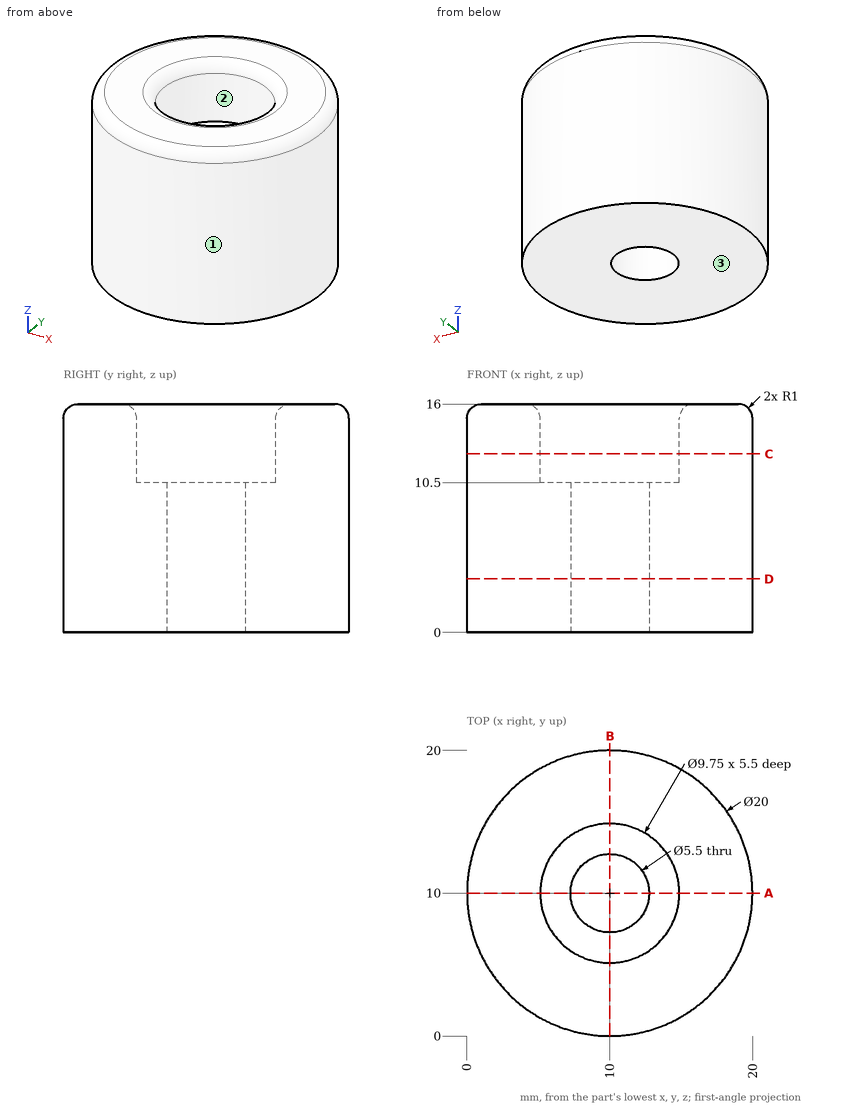
Here's the drawing with two shaded views (mm, measured from the low corner). I have some questions. Coordinates: 2 decimals unless noted, no trailing zeros. Order: outer loops, then holes, each group sorted by start corner. A loop starts at its lowest first (then second) coordinate and runs counter-clockwise, first axis right, second up. Notation, with made-up numbers: (70.5, 51) -> (86.5, 51) arc R19 ccw to (86.5, 85) -> close; hole circle Ø11 at (5, 29.25). An arc over 180 degrees is marked (long way). Write each question's results on one line, items separated by ' | '.
Item 1: I want a section at D-D, the plane z = 3.75. Write out the boundary of the cut face in (x, y), then the cut area to 3 significant figures.
Results are:
outline: circle Ø20 at (10, 10); hole circle Ø5.5 at (10, 10) | area: 290 mm²
Item 2: I want a section at C-C, the plane z = 12.5. Write out the boundary of the cut face in (x, y) (3 decimals), then the cut area to 3 significant figures.
Results are:
outline: circle Ø20 at (10, 10); hole circle Ø9.75 at (10, 10) | area: 239 mm²
Item 3: I want a section at A-A, the plane y = 10. Write out the boundary of the cut face in (x, z) (3 decimals).
Results are:
outline: (0, 0) -> (7.25, 0) -> (7.25, 10.5) -> (5.125, 10.5) -> (5.125, 15) arc R1 ccw to (4.125, 16) -> (1, 16) arc R1 ccw to (0, 15) -> close; (12.75, 0) -> (20, 0) -> (20, 15) arc R1 ccw to (19, 16) -> (15.875, 16) arc R1 ccw to (14.875, 15) -> (14.875, 10.5) -> (12.75, 10.5) -> close
Item 4: If we mould it in two halves opening along Y, with no side actions, what happens to the marked faces 1, 2 and 3? For each: +Y half, -Y half, draft (parallel to the pull), parting line (faces both ways), or undercut.
Results are:
face 1: parting line | face 2: undercut | face 3: draft
Item 5: If I drill on line 1 along Y through (x, z) = (10, 12.5) (3 decimals); line 2 along X through (y, z) = (12.5, 13.5); line 3 along X through (y, z) = (6, 15.25), over which ranges is the centre line in solid material (lowest first)?
Results are:
line 1: 0 to 5.125, 14.875 to 20 | line 2: 0.32 to 5.81, 14.19 to 19.68 | line 3: 0.87 to 7.16, 12.84 to 19.13
Item 6: I'm going to push flat-ended pins straight in: pin 1 Ø8 at (x, y) = (11, 9.5) entering from +Z; pin 2 Ø11 at (x, y) = (10, 10) entering from +Z; pin 3 Ø6 at (y, z) = (6, 8) entering from -X. Where does each tip first touch, or does it pass through?
Results are:
pin 1: z = 15.65 | pin 2: z = 15.93 | pin 3: x = 0.05
